Input: part model. Units: mm. Frame: model coordinates. Face numbers are marked on the shaded views. A direction names the side the tool comes from. Round coordinates to 2 decimals unless told otherwise and drop trailing zeros. Loops run counter-clockwise (first coordinate to the right, second up) from the corner with the lowest first, then second, coordinate; pieces in that order, holes last.
(1) Access query for the marked faces 4, 5 and 6. Directions: +Z, -Z, +X, -X, +Y, -Y. A direction counts if a zero-diameter tool reaches every point of the face in a straight line with its end or side. Return the directions, or none.
(2) Line query: line 1 (Y direction, x = 82, z = -13); line 2 (X direction, y = 67.5, z = 0.5); line 3 (X direction, y = 22.5, z = -6). Output: solid intervals per line, ascending.
(3) Cut plane A-A, the plane x = 0. Output: boundary loops of the cut face in (y, z), and give its area (3 significant figures).
(4) Cut plane B-B, the plane y = 42. Give the number of separate pieces and of enclosed holes in the cut face, and give its area (3 significant figures).
(5) First-contact query: pin 1 Ø1.1 at (x, y) = (96, 58.5) entering from +Z; pin 2 Ø25 at (x, y) = (47, 23.5) entering from -Z; pin 3 Ø5 at (y, z) = (93.5, 10.5) entering from +X; pin 4 Ø3 at (x, z) = (0.5, 13) entering from +Y. Flat tips, straight axial feed; report the tip coordinate or a pass-through.
(6) Draft query along X for the marked faces 1, 2 and 3. Return one class per face: released by +X, released by -X, zero draft, split by the parting line, or undercut.
(7) Cut plane C-C, the plane z = 0. Output: boundary loops of the cut face in (x, y), and give its area (3 significant figures).
(8) Cut plane D-D, the plane y = 137.5. Output: boundary loops of the cut face in (x, z).
Autodesk Inventor part; units mm, degrees
ref_plane "YZ Plane" through (0, 0, 0) normal (1, 0, 0) x (0, 1, 0)
ref_plane "XZ Plane" through (0, 0, 0) normal (0, 1, 0) x (-1, 0, 0)
ref_plane "XY Plane" through (0, 0, 0) normal (0, 0, 1) x (1, 0, 0)
sketch "Sketch1" plane through (0, 0, 0) normal (0, 1, 0) x (-1, 0, 0)
  circle A0 centre (0, 0) radius 15
  line L0 (-17, 0) -> (-91, 0)
  line L1 (-91, 0) -> (-115, 0)
  line L2 (-115, 0) -> (-115, -14.5)
  line L3 (-115, -14.5) -> (-8.8741, -14.5)
  line L4 (-0.35, 0) -> (-0.35, 13.2189)
  line L5 (-9.2718, 14.249) -> (-115, 14.249)
  line L6 (-115, 14.249) -> (-115, -14.5)
  line L7 (-113, -12.5) -> (-11.5217, -12.5)
  line L8 (-113, -12.5) -> (-113, 12.249)
  line L9 (-113, 12.249) -> (-11.7882, 12.249)
  circle A1 centre (0, 0) radius 17
  line L10 (-17, 0) -> (-17, 12.249)
  line L11 (-17, 0) -> (-17, -12.5)
  line L12 (-91, -12.5) -> (-91, 12.249)
  line L13 (-93, -12.5) -> (-93, 12.249)
  line L14 (-17, 12.249) -> (-17, 9.249)
  line L15 (-17, 9.249) -> (-20, 9.249)
  line L16 (-20, 9.249) -> (-20, 12.249)
  line L17 (-20, 12.249) -> (-17, 12.249)
  line L18 (-17, 12.249) -> (-17, 9.249)
  line L19 (-91, 9.249) -> (-88, 9.249)
  line L20 (-88, 9.249) -> (-88, 12.249)
  line L21 (-88, 12.249) -> (-91, 12.249)
  line L22 (-91, 12.249) -> (-91, 9.249)
  line L23 (-17, 9.249) -> (-17, 7.549)
  line L24 (-17, 7.549) -> (-20, 7.549)
  line L25 (-20, 7.549) -> (-20, 4.2225)
  line L26 (-20, 4.2225) -> (-17, 4.2225)
  line L27 (-17, 4.2225) -> (-17, 7.549)
  line L28 (-91, 7.549) -> (-88, 7.549)
  line L29 (-88, 7.549) -> (-88, 4.9725)
  line L30 (-88, 4.9725) -> (-91, 4.9725)
  line L31 (-91, 4.9725) -> (-91, 7.549)
  line L32 (-17, 7.549) -> (-20, 7.549)
  line L33 (-20, 7.549) -> (-20, 9.249)
  line L34 (-20, 9.249) -> (-17, 9.249)
  line L35 (-17, 9.249) -> (-17, 7.549)
  line L36 (-91, 7.549) -> (-88, 7.549)
  line L37 (-88, 7.549) -> (-88, 9.249)
  line L38 (-88, 9.249) -> (-91, 9.249)
  line L39 (-91, 9.249) -> (-91, 7.549)
  line L40 (-91, 7.549) -> (-70.5, 7.549)
  line L41 (-70.5, 7.549) -> (-70.5, 3.549)
  line L42 (-70.5, 3.549) -> (-47.5, 3.549)
  line L43 (-47.5, 3.549) -> (-47.5, -9.451)
  line L44 (-47.5, -9.451) -> (-70.5, -9.451)
  line L45 (-70.5, -9.451) -> (-70.5, 3.549)
  point P0 (-93, 12.249)
  dimension "d0" = 30
  dimension "d1" = 74
  dimension "d2" = 24
  dimension "d3" = 14.5
  dimension "d4" = 29
  dimension "d5" = 2
  dimension "d6" = 2
  dimension "d7" = 2
  dimension "d9" = 2
  dimension "d10" = 3
  dimension "d11" = 3
  dimension "d12" = 3
  dimension "d13" = 1.7
  dimension "d14" = 3
  dimension "d15" = 3
  dimension "d16" = 20.5
  dimension "d17" = 4
  dimension "d18" = 23
  dimension "d19" = 13
extrude "Extrusion1" add sketch "Sketch1" against normal blind 3 contours L11 L7 L12 L0 L45 L44 L43 | L10 L9 A1 | A1 | L0 L43 L42 L41 L40 L37 L20 L9 L16 L33 L25 L26 L10 | A1 L7 L11 | L9 L8 L1 L6 L5 A1 | A1 L3 L2 L1 L8 L7 | L26 L25 L24 L10 | L0 L12 L30 L29 L40 L41 L45 | L10 L15 L16 L9 | L24 L33 L15 L10 | L7 L13 L1 L12 | L1 L13 L9 L12 | L7 L8 L1 L13 | L1 L8 L9 L13 | L12 L28 L29 L30 | L20 L19 L12 L9 | L12 L19 L37 L28
extrude "Extrusion2" add sketch "Sketch1" along normal blind 150 contours A1
extrude "Extrusion3" add sketch "Sketch1" along normal blind 150 contours L10 L9 A1 | A1 L7 L11
extrude "Extrusion4" add sketch "Sketch1" along normal blind 80 contours L9 L8 L1 L6 L5 A1 | A1 L3 L2 L1 L8 L7
extrude "Extrusion5" add sketch "Sketch1" along normal blind 3 contours L24 L33 L15 L10 | L12 L19 L37 L28
extrude "Extrusion6" add sketch "Sketch1" along normal blind 65 contours L26 L25 L24 L10 | L10 L15 L16 L9 | L7 L13 L1 L12 | L1 L13 L9 L12 | L12 L28 L29 L30 | L20 L19 L12 L9
sketch "Sketch2" plane through (0, 65, 0) normal (0, 1, 0) x (1, 0, 0)
  line L0 (113, -12.249) -> (113, 12.5)
  line L1 (113, -12.249) -> (113, -10.999)
  line L2 (113, -10.999) -> (112, -10.999)
  line L3 (112, -10.999) -> (112, -8.999)
  line L4 (112, -8.999) -> (113, -8.999)
  line L5 (113, -12.249) -> (95.4, -12.249)
  line L6 (113, -12.249) -> (17, -12.249)
  line L7 (95.4, -12.249) -> (95.4, -10.999)
  line L8 (95.4, -10.999) -> (96.4, -10.999)
  line L9 (96.4, -10.999) -> (96.4, -8.9987)
  line L10 (96.4, -8.9987) -> (93, -8.9987)
  line L11 (93, -12.249) -> (93, 12.5)
  line L12 (93, -8.9987) -> (93, -12.249)
  line L13 (93, -12.249) -> (95.4, -12.249)
  point P0 (0, 0)
  dimension "d32" = 1.25
  dimension "d33" = 1
  dimension "d34" = 2
  dimension "d35" = 17.6
  dimension "d36" = 1
extrude "Extrusion7" add sketch "Sketch2" along normal up to surface (15 mm away)
extrude "Extrusion8" add sketch "Sketch2" against normal blind 13.5
sketch "Sketch3" plane through (93, 0, -12.5) normal (1, 0, 0) x (0, 0, -1)
  line L0 (-23.499, 51.5) -> (-24.749, 51.5)
  line L1 (-24.749, 51.5) -> (-21.4987, 51.5)
  line L2 (-24.749, 51.5) -> (-21.4987, 51.5)
  line L3 (-24.749, 51.5) -> (-24.749, 48.25)
  line L4 (-24.749, 48.25) -> (-21.4987, 51.5)
  point P0 (-12.5, 0)
  dimension "d44" = 3.25
extrude "Extrusion9" add sketch "Sketch3" along normal up to surface (20 mm away)
sketch "Sketch4" plane through (95.4, 51.5, 12.249) normal (0, 1, 0) x (1, 0, 0)
  line L0 (1, 3.2503) -> (1, 1.25)
  line L1 (17.6, 1.25) -> (16.6, 1.25)
  line L2 (1, 3.2503) -> (16.6, 3.2503)
  line L3 (16.6, 3.2503) -> (16.6, 1.25)
  line L4 (16.6, 1.25) -> (1, 1.25)
  line L5 (1, 1.25) -> (1, 3.2503)
  point P0 (-95.4, 12.249)
extrude "Extrusion10" cut sketch "Sketch4" against normal blind 10
sketch "Sketch5" plane through (17, 80, -12.5) normal (0, 0, 1) x (1, 0, 0)
  line L0 (74, -77) -> (71, -77)
  line L1 (74, -77) -> (74, -61)
  line L2 (74, -80) -> (74, -15)
  line L3 (74, -61) -> (65, -61)
  circle A0 centre (65, -61) radius 3.1
  line L4 (65, -61) -> (65, -49.5)
  line L5 (65, -49.5) -> (65, -38)
  circle A1 centre (65, -49.5) radius 3.1
  circle A2 centre (65, -38) radius 3.1
  circle A3 centre (65, -38) radius 5.1
  circle A4 centre (65, -49.5) radius 5.1
  circle A5 centre (65, -61) radius 5.1
  line L6 (3, -80) -> (71, -80)
  line L7 (64, -80) -> (66, -80)
  line L8 (66, -31.3579) -> (64, -31.3579)
  line L9 (64, -43.001) -> (64, -44.499)
  line L10 (66, -44.499) -> (66, -43.001)
  line L11 (66, -55.999) -> (66, -54.501)
  line L12 (64, -54.501) -> (64, -55.999)
  line L13 (64, -66.001) -> (64, -80)
  line L14 (66, -80) -> (66, -66.001)
  point P0 (-17, -80)
  dimension "d47" = 16
  dimension "d48" = 9
  dimension "d49" = 6.2
  dimension "d50" = 11.5
  dimension "d51" = 11.5
  dimension "d52" = 6.2
  dimension "d53" = 6.2
  dimension "d54" = 2
  dimension "d55" = 2
  dimension "d56" = 2
  dimension "d57" = 2
extrude "Extrusion11" cut sketch "Sketch5" against normal blind 10 contours A0 L4 L3 | L3 L4 A0 | A1 L5 L4 | L4 L5 A1 | A2
properties part number "Open_source_chronograph_main_body_v2"
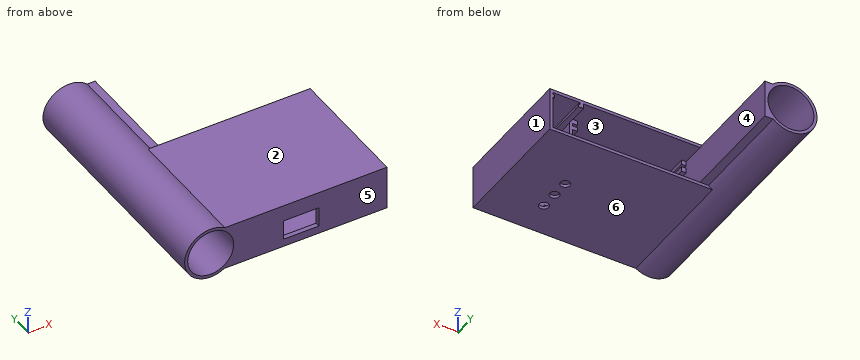
Reported:
1. face 4: +Y
1. face 5: +Z, -Z, +X, -X, -Y
1. face 6: -Z, +X, +Y, -Y
2. line 1: y = -3 to 15.9, 22.1 to 27.4, 33.6 to 38.9, 45.1 to 80
2. line 2: x = -16.99 to -14.99, 14.99 to 17, 113 to 115
2. line 3: x = -15.91 to -13.75, 13.75 to 17, 91 to 93, 113 to 115
3. outline: (-3, -17) - (150, -17) - (150, -15) - (-3, -15) - close; (-3, 15) - (150, 15) - (150, 17) - (-3, 17) - close
3. area: 612 mm2
4. separate pieces: 1
4. enclosed holes: 2
4. area: 782 mm2
5. pin 1: stops at z = 14.25
5. pin 2: stops at z = -14.5
5. pin 3: stops at x = 17
5. pin 4: passes through
6. face 1: released by +X
6. face 2: zero draft
6. face 3: undercut
7. outline: (-17, -3) - (-15, -3) - (-15, 150) - (-17, 150) - close; (15, -3) - (47.5, -3) - (47.5, 0) - (17, 0) - (17, 150) - (15, 150) - close; (70.5, -3) - (115, -3) - (115, 80) - (113, 80) - (113, 0) - (93, 0) - (93, 65) - (91, 65) - (91, 0) - (70.5, 0) - close
7. area: 1,130 mm2
8. outline: (11.52, -12.5) - (17, -12.5) - (17, 12.25) - (11.79, 12.25) arc R17 ccw (long way) to start; hole circle Ø30 at (0, 0)
